Can you work these out from the model? Positions are in its coordinate system, mm. Round coordinates to 2 decimals unless told otherwise and drop trailing zeros. Loops run counter-clockwise (first coordinate to the right, second up) from the corner with the lowest first, then second, coordinate; pieces in that order, holes last.
from build123d import *

# Parameters (mm, degrees)
SKETCH1_R           = 3.9
BOSS_EXTRUDE1_DEPTH = 0.4


with BuildPart() as part:
    # Sketch1 → Boss-Extrude1 (new body)
    with BuildSketch(Plane(origin=(0, 0, 0), x_dir=(1, 0, 0), z_dir=(0, 1, 0))):
        with BuildLine():
            Line((-1.2, 5.521095906), (-1.2, 7.403377608))
            ThreePointArc((-1.2, 7.403377608), (-0.601941834, 7.475805377), (0, 7.5))
            ThreePointArc((0, 7.5), (0.601941834, 7.475805377), (1.2, 7.403377608))
            Line((1.2, 7.403377608), (1.2, 5.521095906))
            ThreePointArc((1.2, 5.521095906), (1.745946018, 5.373469317), (2.274398357, 5.172002718))
            Line((2.274398357, 5.172002718), (3.380775782, 6.694800603))
            ThreePointArc((3.380775782, 6.694800603), (3.907186976, 6.401866129), (4.408389392, 6.067627458))
            ThreePointArc((4.408389392, 6.067627458), (4.881149323, 5.694241063), (5.322416568, 5.284115998))
            Line((5.322416568, 5.284115998), (4.216039143, 3.761318113))
            ThreePointArc((4.216039143, 3.761318113), (4.570946018, 3.320986675), (4.880053845, 2.847380282))
            Line((4.880053845, 2.847380282), (6.670210123, 3.429037316))
            ThreePointArc((6.670210123, 3.429037316), (6.923903162, 2.882631612), (7.132923872, 2.317627458))
            ThreePointArc((7.132923872, 2.317627458), (7.295923674, 1.737670204), (7.41185091, 1.146501677))
            Line((7.41185091, 1.146501677), (5.621694631, 0.564844643))
            ThreePointArc((5.621694631, 0.564844643), (5.65, 0), (5.621694631, -0.564844643))
            Line((5.621694631, -0.564844643), (7.41185091, -1.146501677))
            ThreePointArc((7.41185091, -1.146501677), (7.295923674, -1.737670204), (7.132923872, -2.317627458))
            ThreePointArc((7.132923872, -2.317627458), (6.923903162, -2.882631612), (6.670210123, -3.429037316))
            Line((6.670210123, -3.429037316), (4.880053845, -2.847380282))
            ThreePointArc((4.880053845, -2.847380282), (4.570946018, -3.320986675), (4.216039143, -3.761318113))
            Line((4.216039143, -3.761318113), (5.322416568, -5.284115998))
            ThreePointArc((5.322416568, -5.284115998), (4.881149323, -5.694241063), (4.408389392, -6.067627458))
            ThreePointArc((4.408389392, -6.067627458), (3.907186976, -6.401866129), (3.380775782, -6.694800603))
            Line((3.380775782, -6.694800603), (2.274398357, -5.172002718))
            ThreePointArc((2.274398357, -5.172002718), (1.745946018, -5.373469317), (1.2, -5.521095906))
            Line((1.2, -5.521095906), (1.2, -7.403377608))
            ThreePointArc((1.2, -7.403377608), (0.601941834, -7.475805377), (0, -7.5))
            ThreePointArc((0, -7.5), (-0.601941834, -7.475805377), (-1.2, -7.403377608))
            Line((-1.2, -7.403377608), (-1.2, -5.521095906))
            ThreePointArc((-1.2, -5.521095906), (-1.745946018, -5.373469317), (-2.274398357, -5.172002718))
            Line((-2.274398357, -5.172002718), (-3.380775782, -6.694800603))
            ThreePointArc((-3.380775782, -6.694800603), (-3.907186976, -6.401866129), (-4.408389392, -6.067627458))
            ThreePointArc((-4.408389392, -6.067627458), (-4.881149323, -5.694241063), (-5.322416568, -5.284115998))
            Line((-5.322416568, -5.284115998), (-4.216039143, -3.761318113))
            ThreePointArc((-4.216039143, -3.761318113), (-4.570946018, -3.320986675), (-4.880053845, -2.847380282))
            Line((-4.880053845, -2.847380282), (-6.670210123, -3.429037316))
            ThreePointArc((-6.670210123, -3.429037316), (-6.923903162, -2.882631612), (-7.132923872, -2.317627458))
            ThreePointArc((-7.132923872, -2.317627458), (-7.295923674, -1.737670204), (-7.41185091, -1.146501677))
            Line((-7.41185091, -1.146501677), (-5.621694631, -0.564844643))
            ThreePointArc((-5.621694631, -0.564844643), (-5.65, 0), (-5.621694631, 0.564844643))
            Line((-5.621694631, 0.564844643), (-7.41185091, 1.146501677))
            ThreePointArc((-7.41185091, 1.146501677), (-7.295923674, 1.737670204), (-7.132923872, 2.317627458))
            ThreePointArc((-7.132923872, 2.317627458), (-6.923903162, 2.882631612), (-6.670210123, 3.429037316))
            Line((-6.670210123, 3.429037316), (-4.880053845, 2.847380282))
            ThreePointArc((-4.880053845, 2.847380282), (-4.570946018, 3.320986675), (-4.216039143, 3.761318113))
            Line((-4.216039143, 3.761318113), (-5.322416568, 5.284115998))
            ThreePointArc((-5.322416568, 5.284115998), (-4.881149323, 5.694241063), (-4.408389392, 6.067627458))
            ThreePointArc((-4.408389392, 6.067627458), (-3.907186976, 6.401866129), (-3.380775782, 6.694800603))
            Line((-3.380775782, 6.694800603), (-2.274398357, 5.172002718))
            ThreePointArc((-2.274398357, 5.172002718), (-1.745946018, 5.373469317), (-1.2, 5.521095906))
        make_face()
        with Locations(Location((0, 0, 0), (0, 0, 270))):
            Circle(SKETCH1_R, mode=Mode.SUBTRACT)
    extrude(amount=BOSS_EXTRUDE1_DEPTH)


solid = part.part
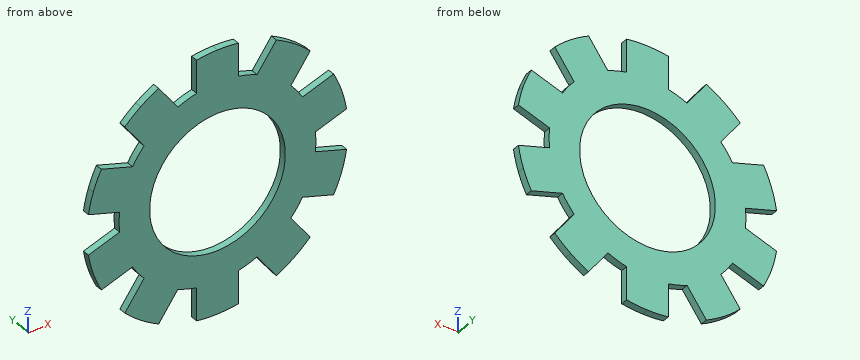
(1) If we section it at B-B, the plane x = -3: List the corners of the cut face in (y, z) for me, then the cut area to 3 significant figures.
Worked answers:
outline: (0, -6.17) - (0.4, -6.17) - (0.4, -2.49) - (0, -2.49) - close; (0, 2.49) - (0.4, 2.49) - (0.4, 6.17) - (0, 6.17) - close
area: 2.94 mm2
(2) Will this pin go through, and if not, where does the flat tip stop? P1, Ø6, axis at x = 0, z = 0, coming from the +Y side.
Worked answers:
P1: passes through
(3) If I drill on line 1 (X direction, y = 0.35, z = 6.5); line 2 (X direction, y = 0.25, z = 0); line 3 (Z direction, x = -5, y = 0.2), over which ranges is the centre line in solid material (lowest first)?
Worked answers:
line 1: x = -3.74 to -3.24, -1.2 to 1.2, 3.24 to 3.74
line 2: x = -5.65 to -3.9, 3.9 to 5.65
line 3: z = -5.59 to -4.84, -2.89 to 2.89, 4.84 to 5.59
(4) If we section it at A-A, the plane z = 0: List the corners of the cut face in (x, y) for me, then the cut area to 3 significant figures.
Worked answers:
outline: (-5.65, 0) - (-3.9, 0) - (-3.9, 0.4) - (-5.65, 0.4) - close; (3.9, 0) - (5.65, 0) - (5.65, 0.4) - (3.9, 0.4) - close
area: 1.40 mm2
